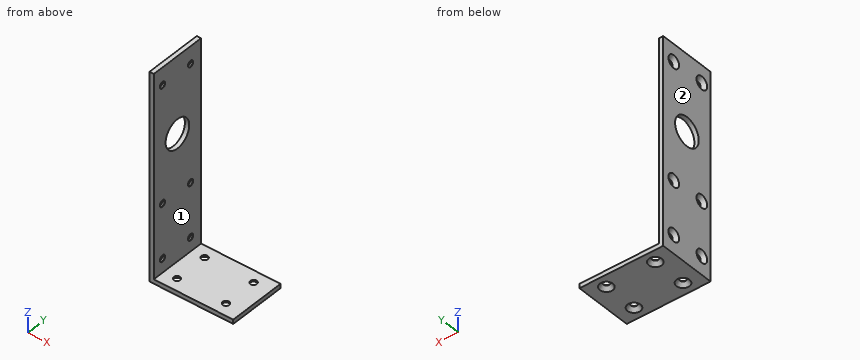
```python
from build123d import *

# Parameters (mm, degrees)
F1_DEPTH       = 40
F3_R           = 10
F4_DEPTH       = 58.001
F6_D           = 4.5
F6_CSINK_D     = 8.96
F6_CSINK_ANGLE = 80
F7_D           = 4.5
F7_CSINK_D     = 8.96
F7_CSINK_ANGLE = 80


# Not quite as in the source:
# - a feature names something its author has since deleted; it is built from what else it names


with BuildPart() as f1:
    # F0 (on Front) → F1 (new body)
    with BuildSketch(Plane.XZ):
        Polygon((3, 143), (0, 143), (0, 0), (58, 0), (58, 3), (3, 3), align=None)
    extrude(amount=F1_DEPTH)

    # F3 (on face) → F4 (cut, through all)
    with BuildSketch(Plane(origin=(0, 0, 0), x_dir=(0, -1, 0), z_dir=(-1, 0, 0))):
        with Locations((20, 90)):
            Circle(F3_R)
    extrude(amount=-F4_DEPTH, mode=Mode.SUBTRACT)

    # F6 (through all)
    with Locations(Plane(origin=(0, 0, 0), x_dir=(0, -1, 0), z_dir=(-1, 0, 0))):
        with Locations((32.6173938811, 50.2130389214), (32.6173938811, 12.7434721217), (8.8956523687, 12.7434721217), (8.8956523687, 49.9434731901), (32.6173938811, 130.9141218662), (8.8956523687, 130.9141218662)):
            CounterSinkHole(F6_D / 2, F6_CSINK_D / 2, counter_sink_angle=F6_CSINK_ANGLE)

    # F7 (through all)
    with Locations(Plane(origin=(0, 0, 0), x_dir=(1, 0, 0), z_dir=(0, 0, -1))):
        with Locations((46.0800911891, 8.2206267661), (12.191168997, 8.2206267661), (12.191168997, 31.5922972435), (46.0800911891, 31.5922972435)):
            CounterSinkHole(F7_D / 2, F7_CSINK_D / 2, counter_sink_angle=F7_CSINK_ANGLE)


solid = f1.part
```
Source: CAD feature listing. Evaluate the final solid. Frame: model axes, mm. Face numbers are marked on the shaded views. A direction names the side the tool comes from. Round coordinates to 2 decimals unless told otherwise and drop trailing zeros. Loops run counter-clockwise (first coordinate to the right, second up) from the corner with the lowest first, then second, coordinate; pieces in that order, holes last. Notation, with made-up numbers: M 23,33 L 48,33 A23 cw 48,42 Z; hole C 25,-20 d8. An arc over 180 degrees is marked long. Use a Markdown table: item, result. Add a question column.
1. Set-up query: the marked faces 1 and 2. Return all of +Z, -Z, +X, -X, +Y, -Y with unobstructed straight access to the full face (end or side cutting, diameter ignored); none if empty.
2. Cut plane C-C, the plane x = 29.5. Output: boundary loops of the cut face in (y, z).
3. Ray query, line 1 along Z through (x, y) = (19.5, -2.5); line 2 along Z through (x, y) = (1.5, -20). Return the intervals inside material, ascending. Write a range as [from, to].
4. Cut plane B-B, the plane z = 82. Output: boundary loops of the cut face in (x, y).
5. Cut plane A-A, the plane y = -20. Output: boundary loops of the cut face in (x, z), and give its area (3 significant figures).
6. Contact query for flat-ended pins moving along their axis: pin 1 (6 mm diameter, centred on y = -8.9, z = 12.74, fed in from -X); pin 2 (10 mm diameter, centred on x = 51, y = -35.5, fed in from +Z); pin 3 (20 mm diameter, centred on y = -20, z = 61, fed in from +X); pin 4 (2.5 mm diameter, centred on y = -8.9, z = 130.91, fed in from +X). Output: stop coordinate, or through.
Solution:
| question | item | result |
|---|---|---|
| 1 | face 1 | +Z, +X, +Y, -Y |
| 1 | face 2 | +Z, -Z, -X, +Y, -Y |
| 2 | outline | M -40,0 L 0,0 L 0,3 L -40,3 Z |
| 3 | line 1 | z = [0, 3] |
| 3 | line 2 | z = [0, 80], [100, 143] |
| 4 | outline | M 0,-40 L 3,-40 L 3,-26 L 0,-26 Z; M 0,-14 L 3,-14 L 3,0 L 0,0 Z |
| 5 | outline | M 0,0 L 58,0 L 58,3 L 3,3 L 3,80 L 0,80 Z; M 0,100 L 3,100 L 3,143 L 0,143 Z |
| 5 | area | 534 mm2 |
| 6 | pin 1 | stops at x = 1.76 |
| 6 | pin 2 | stops at z = 3 |
| 6 | pin 3 | stops at x = 3 |
| 6 | pin 4 | passes through |
